Model file for the job. Use its own axes, mm. A direction names the side the tool comes from. Round coordinates to 2 decimals unless told otherwise and drop trailing zeros. Use CSV: the item, a comma, the result in double quotes.
```python
from build123d import *

# Parameters (mm, degrees)
SKETCH3_R               = 29.972
SKETCH3_R_2             = 19.05
SKETCH6_W               = 49.478831
SKETCH6_H               = 30.48
CUT_EXTRUDE2_DEPTH      = 93.970246
CUT_EXTRUDE3_DEPTH      = 93.970246
CUT_EXTRUDE3_DEPTH_BACK = 2.54
SKETCH7_W               = 63.5
SKETCH7_H               = 6.35
SKETCH8_R               = 43.612232
CUT_EXTRUDE4_DEPTH      = 103.320343


with BuildPart() as part:
    # Sketch1 → Revolve1 (revolve)
    with BuildSketch(Plane.XY, mode=Mode.PRIVATE) as revolve1_sk:
        Polygon((-62.23, -29.972), (-26.67, -29.972), (-26.67, -24.0538), (-62.23, -24.2824), align=None)
    revolve(revolve1_sk.sketch.rotate(Axis((-62.23, 0, 0), (1, 0, 0)), 270), axis=Axis((-62.23, 0, 0), (1, 0, 0)))


with BuildPart() as body_2:
    # Sketch2 → Revolve2 (revolve)
    with BuildSketch(Plane.XY, mode=Mode.PRIVATE) as revolve2_sk:
        Polygon((24.2824, 62.23), (24.0538, 26.67), (29.972, 26.67), (29.972, 62.23), align=None)
    revolve(revolve2_sk.sketch.rotate(Axis((0, 0, 0), (0, 1, 0)), 90), axis=Axis((0, 0, 0), (0, 1, 0)))


with BuildPart() as sweep1_tool:
    # Sweep1: sweep along a path in Sketch4
    with BuildLine(Plane.XY) as sweep1_path:
        ThreePointArc((-26.67, 0), (-7.811462, 7.811462), (0, 26.67))
    # Sketch3 → Sweep1 (sweep)
    with BuildSketch(Plane(origin=(-26.67, 0, 0), x_dir=(0, 0, -1), z_dir=(1, 0, 0))):
        Circle(SKETCH3_R)
        Circle(SKETCH3_R_2, mode=Mode.SUBTRACT)
    sweep(path=sweep1_path.line)


with BuildPart() as part_1:
    add(part.part)


with BuildPart() as part_2:
    # Sweep1: joined with sweep1_tool
    add(part_1.part.fuse(sweep1_tool.part, body_2.part, tol=0.00001))

    # Sketch6 → Cut-Extrude2 (cut, through all)
    with BuildSketch(Plane.XY):
        with Locations((-54.863748, 0)):
            Rectangle(SKETCH6_W, SKETCH6_H)
    extrude(amount=-CUT_EXTRUDE2_DEPTH, mode=Mode.SUBTRACT)

    # Sketch7 → Cut-Extrude3 (cut, two sides: drawn at the far end of the back side and taken through both)
    with BuildSketch(Plane(origin=(0, 0, 0), x_dir=(0, 0, -1), z_dir=(1, 0, 0)).offset(-CUT_EXTRUDE3_DEPTH_BACK)):
        with Locations((0, 42.3418)):
            Rectangle(SKETCH7_W, SKETCH7_H)
    extrude(amount=CUT_EXTRUDE3_DEPTH + CUT_EXTRUDE3_DEPTH_BACK, mode=Mode.SUBTRACT)

    # Sketch8 → Cut-Extrude4 (cut, through all)
    with BuildSketch(Plane.XZ.offset(-45.5168)):
        Circle(SKETCH8_R)
    extrude(amount=-CUT_EXTRUDE4_DEPTH, mode=Mode.SUBTRACT)


solid = part_2.part
```
Q1. Which spindle directions (+Z, -Z, +X, -X, +Y, -Y) get a long thin tool onto all of the face, cutting with end or side? Do faces 1 (the flat face through (-46, -15.24, -22)), 2 (the flat face through (-26.67, -7, 18)), 3 (the flat face through (-2.54, 42, 27)), 4 (the flat face through (-24.4, 45.517, 0.1)), 5 (the conical face through (-23.9, 33.9, 3.1)). Say none if no direction does.
From the geometry:
face 1,"-Z, -X"
face 2,"-X"
face 3,"+Z, -Z, +X, +Y"
face 4,"+Z, -Z, +X, -X, +Y"
face 5,"+Y"
Q2. Pin check, flat tips, straight feed: pin 1 (3 mm diameter, centred on x = -30.5, y = 12.5, fed in from -Z); pin 2 (2 mm diameter, centred on x = -14, z = 11.5, fed in from +Y); pin 3 (5 mm diameter, centred on x = 6.5, z = -22, fed in from -Y). Stop position of each tip, or through.
From the geometry:
pin 1,"stops at z = -27.86"
pin 2,"stops at y = 26.67"
pin 3,"stops at y = -10.71"
Q3. Mould opens along Z. For faces 6 (the cylindrical face through (-25.273, 34.131, -16.113)), 7 (the flat face through (-2.54, 42, -27)), 8 (the conical face through (-44.699, -7.26, 23.054)), 9 (the flat face through (-7, 26.67, -18)) say: +Z half, -Z half, draft (parallel to the pull), parting line (faces both ways), or undercut.
From the geometry:
face 6,"parting line"
face 7,"draft"
face 8,"undercut"
face 9,"undercut"
Q4. Probe line 1 along X through (y, z) = (37, 1.5); line 2 along Z through (x, y) = (-53, 21); line 3 along Y through (x, z) = (-30.5, -20.5). List the from-to ranges inside material, lowest first.
From the geometry:
line 1,"x = -29.93 to -24.07, 24.07 to 29.93"
line 2,"z = -21.39 to -12.07, 12.07 to 21.39"
line 3,"y = -21.86 to -15.24, 15.24 to 21.86"
